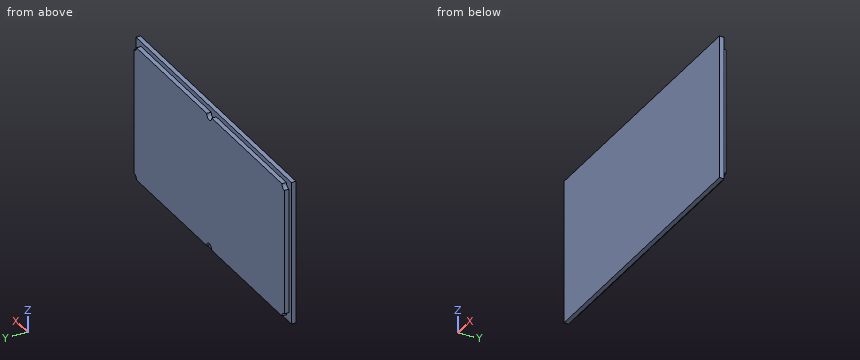
```python
from build123d import *

# Parameters (mm, degrees)
SKETCH3_7_W         = 128
SKETCH3_7_H         = 64
BOSS_EXTRUDE4_DEPTH = 2
BOSS_EXTRUDE6_DEPTH = 4


with BuildPart() as part:
    # Sketch3<7> → Boss-Extrude4 (new body)
    with BuildSketch(Plane(origin=(0, 0, 0), x_dir=(1, 0, 0), z_dir=(0, 1, 0))):
        with Locations((0, -104)):
            Rectangle(SKETCH3_7_W, SKETCH3_7_H)
        with BuildLine():
            Line((-2.097617696, -74.1), (-59.902382304, -74.1))
            ThreePointArc((-59.902382304, -74.1), (-60.51507576, -75.48492424), (-61.9, -76.097617696))
            Line((-61.9, -76.097617696), (-61.9, -131.902382304))
            ThreePointArc((-61.9, -131.902382304), (-60.51507576, -132.51507576), (-59.902382304, -133.9))
            Line((-59.902382304, -133.9), (-2.097617696, -133.9))
            ThreePointArc((-2.097617696, -133.9), (0, -131.9), (2.097617696, -133.9))
            Line((2.097617696, -133.9), (59.902382304, -133.9))
            ThreePointArc((59.902382304, -133.9), (60.51507576, -132.51507576), (61.9, -131.902382304))
            Line((61.9, -131.902382304), (61.9, -76.097617696))
            ThreePointArc((61.9, -76.097617696), (60.51507576, -75.48492424), (59.902382304, -74.1))
            Line((59.902382304, -74.1), (2.097617696, -74.1))
            ThreePointArc((2.097617696, -74.1), (0, -76.1), (-2.097617696, -74.1))
        make_face(mode=Mode.SUBTRACT)
    extrude(amount=BOSS_EXTRUDE4_DEPTH)

    # Sketch3 → Boss-Extrude6 (add)
    with BuildSketch(Plane(origin=(0, 0, 0), x_dir=(1, 0, 0), z_dir=(0, 1, 0))):
        with BuildLine():
            Line((-61.9, -76.097617696), (-61.9, -131.902382304))
            ThreePointArc((-61.9, -131.902382304), (-60.51507576, -132.51507576), (-59.902382304, -133.9))
            Line((-59.902382304, -133.9), (-2.097617696, -133.9))
            ThreePointArc((-2.097617696, -133.9), (0, -131.9), (2.097617696, -133.9))
            Line((2.097617696, -133.9), (59.902382304, -133.9))
            ThreePointArc((59.902382304, -133.9), (60.51507576, -132.51507576), (61.9, -131.902382304))
            Line((61.9, -131.902382304), (61.9, -76.097617696))
            ThreePointArc((61.9, -76.097617696), (60.51507576, -75.48492424), (59.902382304, -74.1))
            Line((59.902382304, -74.1), (2.097617696, -74.1))
            ThreePointArc((2.097617696, -74.1), (0, -76.1), (-2.097617696, -74.1))
            Line((-2.097617696, -74.1), (-59.902382304, -74.1))
            ThreePointArc((-59.902382304, -74.1), (-60.51507576, -75.48492424), (-61.9, -76.097617696))
        make_face()
    extrude(amount=BOSS_EXTRUDE6_DEPTH)


solid = part.part
```
Part model, mm, in its own coordinate system. Coordinates: 2 decimals unless noted, no trailing zeros. Order: outer loops, then holes, each group sorted by start corner. A loop starts at its lowest first (then second) coordinate and runs counter-clockwise, first axis right, second up. Notation, with made-up numbers: (20, 2.25) -> (51, 2.25) arc R24 cw to (51, 30.25) -> close; hole circle Ø4 at (79, 24.25). An arc over 180 degrees is marked (long way). Put each result on its own line as item: value. Start each with the question number.
(1) Band-saw the part on A-A (x = -32.5). Give the cut face in (y, z), then the cut area to 3 significant figures.
(2) Pin check, flat tips, straight feed: pin 1 Ø1.5 at (x, z) = (-50.5, 86.5) entering from -Y; pin 2 Ø1 at (y, z) = (3, 80) entering from +X; pin 3 Ø1.6 at (x, y) = (43, 3) entering from -Z. Stop position of each tip, or through.
(3) Band-saw the part on C-C (y = 2.65). Give the cut face in (x, z), then the cut area to 3 significant figures.
(4) Band-saw the part on B-B (z = 77.5). Give the cut face in (x, y).
(5) Probe line 1 along X through (y, z) = (2.8, 76.5); line 2 along Z through (x, y) = (-3.5, 3.35); line 3 along Z through (x, y) = (1, 3.25). List the from-to ranges inside material, lowest first. Write a range as [from, to].
Determined:
1. outline: (0, 72) -> (2, 72) -> (2, 74.1) -> (4, 74.1) -> (4, 133.9) -> (2, 133.9) -> (2, 136) -> (0, 136) -> close
1. area: 248 mm²
2. pin 1: stops at y = 0
2. pin 2: stops at x = 61.9
2. pin 3: stops at z = 74.1
3. outline: (-61.9, 76.1) arc R2.1 cw to (-59.9, 74.1) -> (-2.1, 74.1) arc R2.1 cw to (2.1, 74.1) -> (59.9, 74.1) arc R2.1 cw to (61.9, 76.1) -> (61.9, 131.9) arc R2.1 cw to (59.9, 133.9) -> (2.1, 133.9) arc R2.1 cw to (-2.1, 133.9) -> (-59.9, 133.9) arc R2.1 cw to (-61.9, 131.9) -> close
3. area: 7,380 mm²
4. outline: (-64, 0) -> (64, 0) -> (64, 2) -> (61.9, 2) -> (61.9, 4) -> (-61.9, 4) -> (-61.9, 2) -> (-64, 2) -> close
5. line 1: x = [-61.9, 61.9]
5. line 2: z = [74.1, 133.9]
5. line 3: z = [75.85, 132.15]
